Design review of the part shown in the three views and the two pictorial views. Dimensions are in mm from the part's minimum x, y and z. A direction names the side the tool comes from. Give positions to 0.01 mm unless a question says otherwise; leave off trailing zeros. Write each loop counter-clockwise with the first axis right and the second up, starting at its lowest first coordinate (ties: lowest second). Pieces come first, ordered by that corner, then holes. Notation, with made-up numbers: M 20,85.25 L 66,85.25 A26 ccw 66,119.25 Z; hole C 60.25,69 d2. An arc over 180 degrees is marked long. Write item = value, one per line.
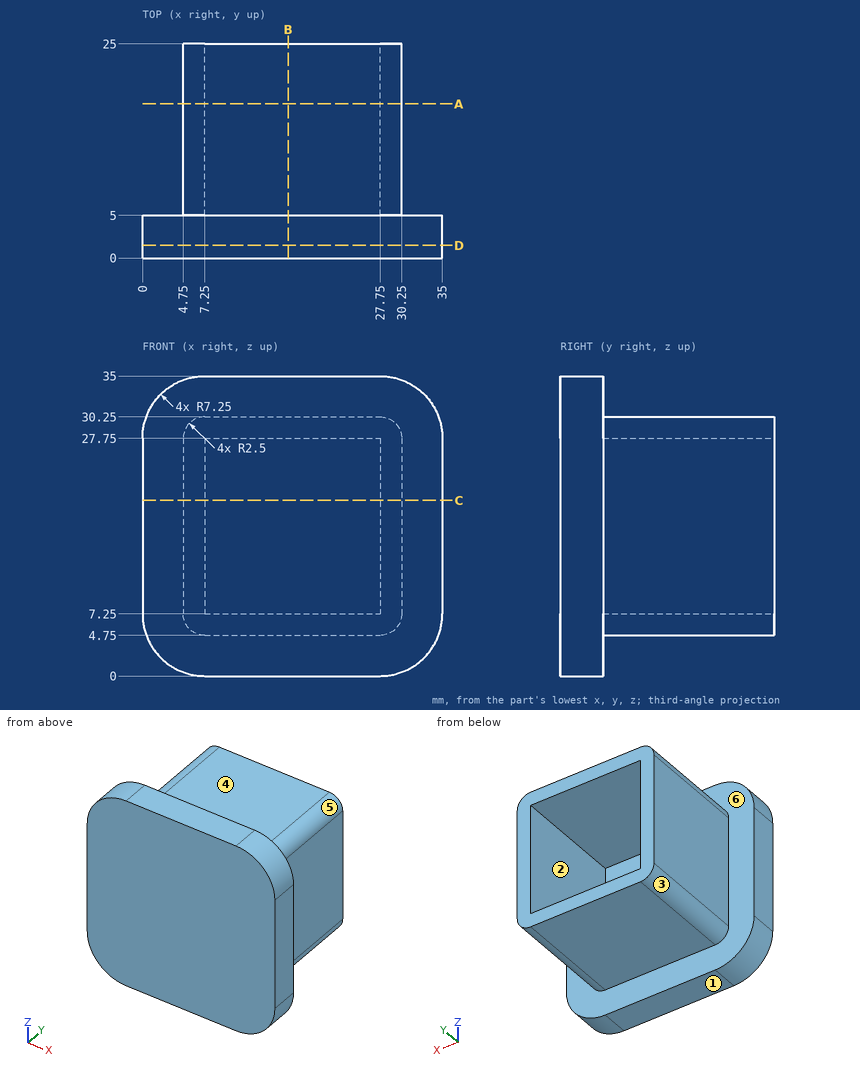
1. Machinability: for the marked faces 4, 5 and 6, which of the approach directions +Z, -Z, +X, -X, +Y, -Y give a long, thin tool a straight path to every point of the face, cutting with its end or side? Answer none if there is none.
Responses:
face_4 = +Z, +X, -X, +Y
face_5 = +Z, +X, +Y
face_6 = +Y
2. We need section A-A, the plane y = 18. Write out the cut boundary in (x, z), then the cut area to 3 significant figures.
Responses:
outline = M 4.75,7.25 A2.5 ccw 7.25,4.75 L 27.75,4.75 A2.5 ccw 30.25,7.25 L 30.25,27.75 A2.5 ccw 27.75,30.25 L 7.25,30.25 A2.5 ccw 4.75,27.75 Z; hole M 7.25,7.25 L 27.75,7.25 L 27.75,27.75 L 7.25,27.75 Z
area = 225 mm2
3. Insertion check: P1, Ø8, axis at x = 26.5, y = 17, coming from the +Z side; P2, Ø2, axis at y = 11, z = 26, coming from the -X side; P3, Ø10, axis at y = 15.5, z = 21.5, coming from the +X side. Each pin has a flat end and moves straight along its axis. Give the tip position at first contact, or say it passes through.
Responses:
P1 = 30.25
P2 = 4.75
P3 = 30.25
4. For line 1 along Z through (x, y) = (12, 13); line 2 along Y through (x, z) = (5, 6), list the stretches that pass through material, from the lowest coordinate up. Write a range as from..to.
Responses:
line_1 = 4.75..7.25, 27.75..30.25
line_2 = 0..5
5. We need section B-B, the plane x = 17. Write out the cut boundary in (y, z).
Responses:
outline = M 0,0 L 5,0 L 5,4.75 L 25,4.75 L 25,7.25 L 5,7.25 L 5,27.75 L 25,27.75 L 25,30.25 L 5,30.25 L 5,35 L 0,35 Z
6. We need section D-D, the plane y = 1.5. Write out the cut boundary in (x, z), then the cut area to 3 significant figures.
Responses:
outline = M 0,7.25 A7.25 ccw 7.25,0 L 27.75,0 A7.25 ccw 35,7.25 L 35,27.75 A7.25 ccw 27.75,35 L 7.25,35 A7.25 ccw 0,27.75 Z
area = 1,180 mm2
7. The part is to be moulded in two halves that separate along X. For the marked faces 1, 2 and 3, say which applies: +X half, -X half, draft (parallel to the pull), parting line (faces both ways), or undercut.
Responses:
face_1 = draft
face_2 = undercut
face_3 = -X half
8. We need section C-C, the plane z = 20.5. Write out the cut boundary in (x, y).
Responses:
outline = M 0,0 L 35,0 L 35,5 L 30.25,5 L 30.25,25 L 27.75,25 L 27.75,5 L 7.25,5 L 7.25,25 L 4.75,25 L 4.75,5 L 0,5 Z
